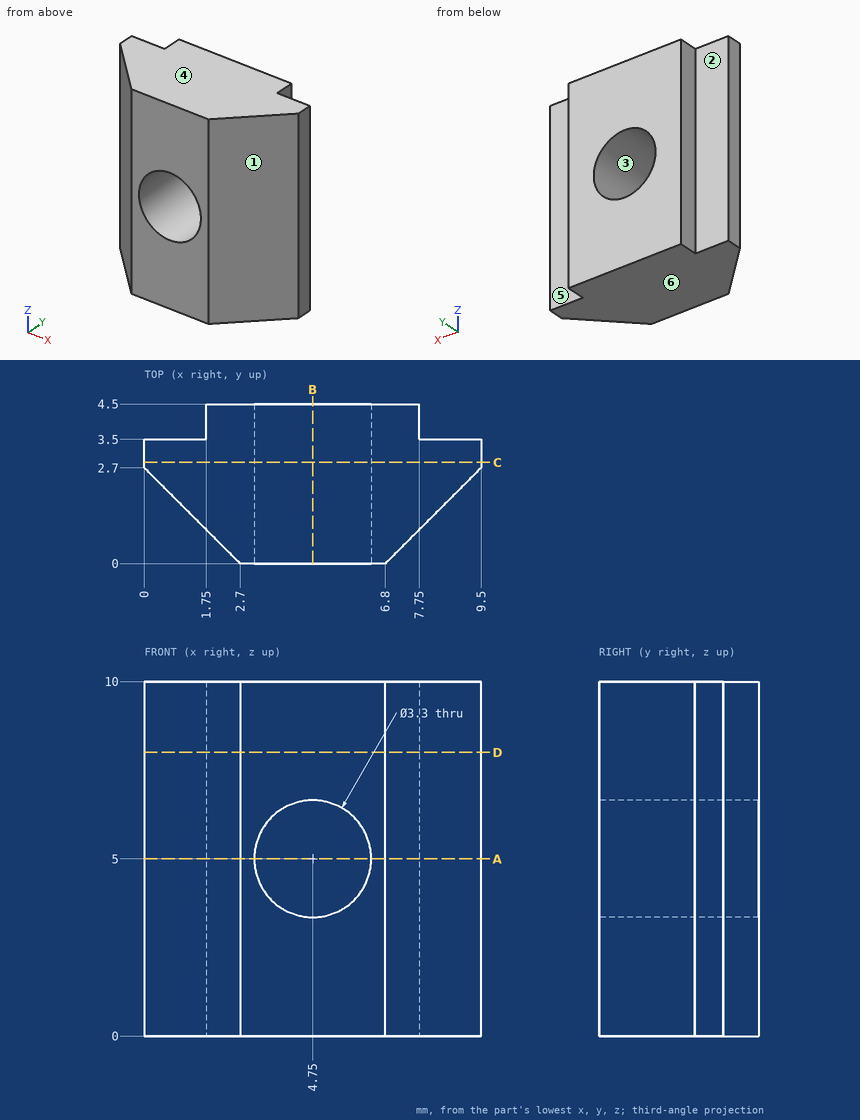
Geometry: see drawing. Coordinates: mm, zero at the bounding-box minimum. A direction names the side the tool comes from. Round coordinates to 2 decimals unless told otherwise and drop trailing zeros. Loops run counter-clockwise (first coordinate to the right, second up) from the corner with the lowest first, then second, coordinate; pieces in that order, holes last. Notation, with made-up numbers: (-30, 46.5) - (24, 46.5) arc R13 ccw to (24, 57.5) - close; hole circle Ø11 at (2.5, -36). An arc over 180 degrees is marked (long way). One line per item, written item: value. Start each with the question number.
(1) Access query for the marked faces 1 and 2. Directions: +Z, -Z, +X, -X, +Y, -Y. A direction counts if a zero-diameter tool reaches every point of the face in a straight line with its end or side. Return the directions, or none.
(2) Ray query, line 1 (Z direction, x = 4.75, y = 3.2); line 2 (X direction, y = 3, z = 5); line 3 (X direction, y = 4.25, z = 2.75). Return the intervals inside material, ascending. Write a range as [from, to].
(3) Section D-D, the plane z = 8. Return loops of the section in (x, y).
(4) Section C-C, the plane y = 2.85. Return loops of the section in (x, z), plus the area to 3 significant figures.
(5) Section B-B, the plane x = 4.75. Return loops of the section in (y, z).
(6) Contact query for flat-ended pins moving along their axis: P1, Ø0.8, axis at y = 4, z = 6.5, coming from the -X side; P2, Ø2.5, axis at x = 4.75, z = 5, coming from the -Y side; P3, Ø0.5, axis at x = 1, z = 3, coming from the +Y side. Output: stop coordinate, or through.
(7) Draft query along Z for the marked faces 3, 4, 5 and 6. Return one class per face: +Z half, -Z half, draft (parallel to the pull), parting line (faces both ways), or undercut.
(8) Section A-A, the plane z = 5. Return loops of the section in (x, y), plus the area to 3 significant figures.
Results below:
1. face 1: +Z, -Z, +X, -Y
1. face 2: +Z, -Z, -X, +Y
2. line 1: [0, 3.35], [6.65, 10]
2. line 2: [0, 3.1], [6.4, 9.5]
2. line 3: [1.75, 7.75]
3. outline: (0, 2.7) - (2.7, 0) - (6.8, 0) - (9.5, 2.7) - (9.5, 3.5) - (7.75, 3.5) - (7.75, 4.5) - (1.75, 4.5) - (1.75, 3.5) - (0, 3.5) - close
4. outline: (0, 0) - (9.5, 0) - (9.5, 10) - (0, 10) - close; hole circle Ø3.3 at (4.75, 5)
4. area: 86.4 mm^2
5. outline: (0, 0) - (4.5, 0) - (4.5, 3.35) - (0, 3.35) - close; (0, 6.65) - (4.5, 6.65) - (4.5, 10) - (0, 10) - close
6. P1: x = 1.75
6. P2: through
6. P3: y = 3.5
7. face 3: undercut
7. face 4: +Z half
7. face 5: draft
7. face 6: -Z half
8. outline: (0, 2.7) - (2.7, 0) - (3.1, 0) - (3.1, 4.5) - (1.75, 4.5) - (1.75, 3.5) - (0, 3.5) - close; (6.4, 0) - (6.8, 0) - (9.5, 2.7) - (9.5, 3.5) - (7.75, 3.5) - (7.75, 4.5) - (6.4, 4.5) - close
8. area: 17.1 mm^2
